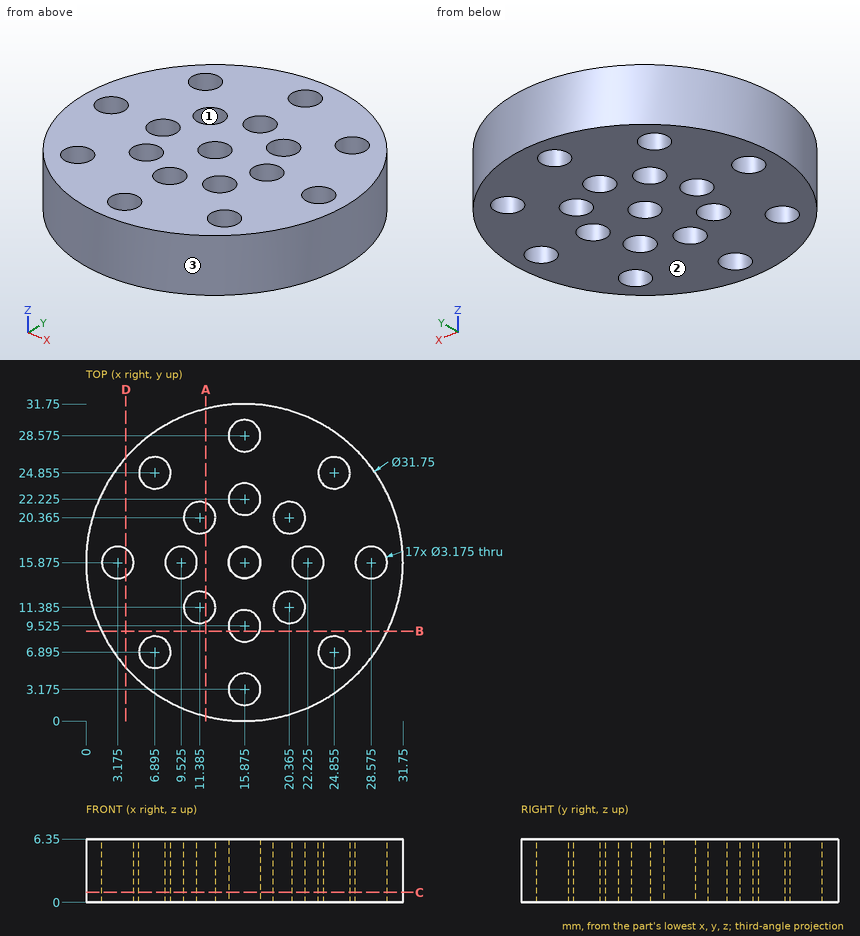
Design review of the part shown in the three views and the two pictorial views. Dimensions are in mm from the part's minimum x, y and z. Round coordinates to 2 decimals unless told otherwise and drop trailing zeros. Write each loop counter-clockwise with the first axis right and the second up, starting at its lowest first coordinate (ties: lowest second). Pieces come first, ordered by that corner, then holes. Notation, with made-up numbers: M 68,-0.5 L 126,-0.5 A22 ccw 126,21.5 Z; hole C -6.75,46.25 d3. An arc over 180 degrees is marked long. One line per item, written item: value. Start each with the question number.
1. Take a section at B-B on y = 9. State the section outline as (x, z) points, then the cut area to 3 significant figures.
2. Take a section at C-C on z = 1. State how many separate pieces and enclosed holes the cut face has, then the cut area to 3 significant figures.
3. Take a section at A-A on x = 12. State the section outline as (y, z) points, then the cut area to 3 significant figures.
4. Clearance check with flat-ended pins moving along their axes: P1, Ø1.5, axis at y = 9, z = 5.5, coming from the -X side; P2, Ø3.5, axis at x = 24.86, y = 6.89, coming from the -Z side; P3, Ø1, axis at x = 14.5, z = 3.5, coming from the -Y side; P4, Ø1, axis at y = 17.5, z = 5, coming from the +X side. State where each tip first meets the part, or that it passes through.
5. To check wall thickness, follow probe 1 along Y at (x, z) = (23.5, 1.5); probe 2 along X at (y, z) = (19.5, 4) (1 decimal); probe 3 along Y at (x, z) = (15.5, 5) (1 decimal). State the ranges of each line that lie inside material, in increasing order. Write a range as from..to.
6. Take a section at D-D on x = 4. State the section outline as (y, z) points.
7. Draft analysis for pull direction X (two halves, no side actions). For the marked faces 1, 2 and 3, state which applies: pulls with the +X half, pulls with the -X half, needs draft (parallel to the pull), parting line crosses it, or undercut.
Computed:
1. outline: M 1.57,0 L 14.38,0 L 14.38,6.35 L 1.57,6.35 Z; M 17.37,0 L 30.18,0 L 30.18,6.35 L 17.37,6.35 Z
1. area: 163 mm²
2. separate pieces: 1
2. enclosed holes: 17
2. area: 657 mm²
3. outline: M 0.48,0 L 9.92,0 L 9.92,6.35 L 0.48,6.35 Z; M 12.85,0 L 18.9,0 L 18.9,6.35 L 12.85,6.35 Z; M 21.83,0 L 31.27,0 L 31.27,6.35 L 21.83,6.35 Z
3. area: 158 mm²
4. P1: stops at x = 1.23
4. P2: stops at z = 0
4. P3: stops at y = 0.02
4. P4: stops at x = 31.71
5. probe 1: y = 1.95..6.07, 7.72..14.93, 16.82..24.03, 25.68..29.8
5. probe 2: x = 0.4..10.1, 12.7..19, 21.7..31.3
5. probe 3: y = 0..1.6, 4.7..8, 11.1..14.3, 17.4..20.7, 23.8..27, 30.1..31.7
6. outline: M 5.34,0 L 14.52,0 L 14.52,6.35 L 5.34,6.35 Z; M 17.23,0 L 26.41,0 L 26.41,6.35 L 17.23,6.35 Z
7. face 1: undercut
7. face 2: needs draft
7. face 3: parting line crosses it
